Here's how the part is built. I have some questions about the finished solid (model axes, mm). Coordinates: 2 decimals unless noted, no trailing zeros. Write each loop counter-clockwise with the first axis right and the second up, starting at its lowest first coordinate (ties: lowest second). Pieces come first, ordered by that corner, then holes. Notation, with made-up numbers: (81, 49.5) -> (105, 49.5) arc R28 ccw to (105, 84.5) -> close; hole circle Ø8 at (77, 84). An arc over 180 degrees is marked (long way). Put each result on its own line as item: value. Start each with the question number.
Item 1: I want a section at A-A, the plane x = 0. List the corners of the cut face in (y, z) for me.
Item 2: I want a section at C-C, the plane z = 21.5. List the corners of the cut face in (x, y) for me.
Item 3: For pin 1 (2 mm diameter, centred on y = 126, z = -2.5, fed in from +X); pin 2 (10 mm diameter, centred on x = 0.5, y = 135.5, fed in from +Z); pin 3 (10 mm diameter, centred on x = 19.5, y = 19, fed in from -Z); pin 4 (6 mm diameter, centred on x = 22.5, y = 103.5, fed in from +Z), each with a flat end and sliding along its axis, tell me the tip position at first contact or that it passes through.
Item 4: I need wall thicknesses on line 1 (Z direction, x = 1, y = 10.5); line 2 (Z direction, x = 20, y = 108); line 3 (Y direction, x = 19.5, z = -18.5). Which ranges of each line are inside material? Lowest first, please. Write a range as [from, to].
Item 5: I want a section at B-B, the plane y = 123. List the corners of the cut face in (x, z) for me.
from build123d import *

# Parameters (mm, degrees)
CROQUIS1_R              = 31.75
SALIENTE_EXTRUIR1_DEPTH = 170
CORTAR_EXTRUIR1_DEPTH   = 90
SALIENTE_EXTRUIR2_DEPTH = 8


with BuildPart() as part:
    # Croquis1 → Saliente-Extruir1 (new body)
    with BuildSketch(Plane(origin=(0, 0, 0), x_dir=(1, 0, 0), z_dir=(0, 1, 0))):
        with Locations(Location((0, 0, 0), (0, 0, 270))):
            Circle(CROQUIS1_R)
    extrude(amount=SALIENTE_EXTRUIR1_DEPTH)

    # Croquis2 → Cortar-Extruir1 (cut, symmetric)
    with BuildSketch(Plane.XY):
        Polygon((-31.75, 170), (31.75, 160), (31.75, 170), align=None)
    extrude(amount=CORTAR_EXTRUIR1_DEPTH, both=True, mode=Mode.SUBTRACT)

    # Croquis3 → Saliente-Extruir2 (add)
    with BuildSketch(Plane.XZ):
        Polygon((-31.75, 0), (-31.75, 2), (-28.75, 2), (-28.75, -2), (-31.75, -2), align=None)
    extrude(amount=-SALIENTE_EXTRUIR2_DEPTH)


solid = part.part
Calculated:
1. outline: (0, -31.75) -> (165, -31.75) -> (165, 31.75) -> (0, 31.75) -> close
2. outline: (-23.36, 0) -> (23.36, 0) -> (23.36, 161.32) -> (-23.36, 168.68) -> close
3. pin 1: stops at x = 31.71
3. pin 2: stops at z = 31.75
3. pin 3: stops at z = -28.25
3. pin 4: stops at z = 25.06
4. line 1: z = [-31.73, 31.73]
4. line 2: z = [-24.66, 24.66]
4. line 3: y = [0, 161.93]
5. outline: circle Ø63.5 at (0, 0)
